```python
from build123d import *

# Parameters (mm, degrees)
SKETCH1_R           = 31.75
SKETCH1_R_2         = 29.21
BOSS_EXTRUDE1_DEPTH = 12.7
SKETCH2_W           = 76.2
SKETCH2_H           = 76.2
BOSS_EXTRUDE2_DEPTH = 2.54
FILLET1_R           = 6.35


with BuildPart() as part:
    # Sketch1 → Boss-Extrude1 (new body)
    with BuildSketch(Plane(origin=(0, 0, 0), x_dir=(1, 0, 0), z_dir=(0, 1, 0))):
        with Locations(Location((0, 0, 0), (0, 0, 270))):
            Circle(SKETCH1_R)
        with Locations(Location((0, 0, 0), (0, 0, 270))):
            Circle(SKETCH1_R_2, mode=Mode.SUBTRACT)
    extrude(amount=BOSS_EXTRUDE1_DEPTH)

    # Sketch2 → Boss-Extrude2 (add)
    with BuildSketch(Plane(origin=(0, 0, 0), x_dir=(1, 0, 0), z_dir=(0, 1, 0))):
        Rectangle(SKETCH2_W, SKETCH2_H)
    extrude(amount=BOSS_EXTRUDE2_DEPTH)

    # Fillet1
    fillet1_edges = [part.edges().sort_by_distance(p)[0] for p in [
        (38.1, 1.27, 38.1),
        (38.1, 1.27, -38.1),
        (-38.1, 1.27, -38.1),
        (-38.1, 1.27, 38.1),
    ]]
    fillet(fillet1_edges, radius=FILLET1_R)


solid = part.part
```
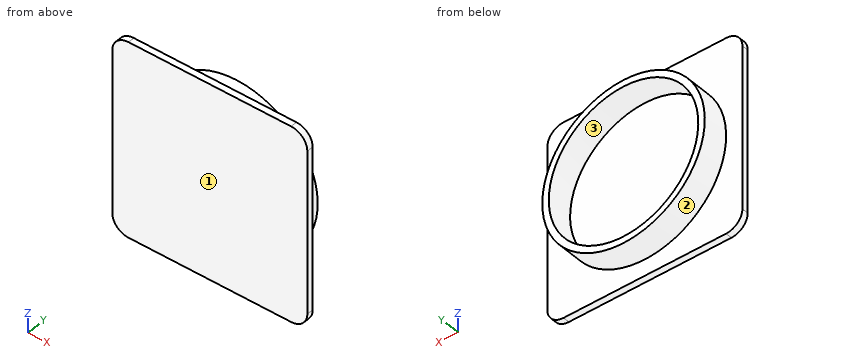
The model under review builds one solid part; all positions refer to its coordinate system, in mm. Face numbers are marked on the shaded views. Round coordinates to 2 decimals unless told otherwise and drop trailing zeros. Loops run counter-clockwise (first coordinate to the right, second up) from the corner with the lowest first, then second, coordinate; pieces in that order, holes last. Notation, with made-up numbers: (84, 75) - (105, 75) arc R17 cw to (105, 100) - close; hole circle Ø2 at (14.25, -36). An arc over 180 degrees is marked (long way). Use a Markdown table: item, result. Add a question column.
Q1. Insertion check: pin 1 Ø2 at (x, z) = (18.5, 0) entering from +Y; pin 2 Ø3 at (y, z) = (6.5, 1) entering from +X. Each pin has a flat end and moves straight along its axis. Give the tip position at first contact, or say it passes through.
Q2. Add section C-C (y = 6.5). State the section outline as (x, z) points, plus the area to 3 significant figures.
Q3. For probe 1 along X at (y, z) = (9, 0); probe 2 along Y at (x, z) = (-19.5, -3), list the stretches that pass through material, from the lowest coordinate up.
Q4. Add section A-A (x = 0). State the section outline as (y, z) points, plus the area to 3 significant figures.
Q5. The part is to be moulded in two halves that separate along Z. For the marked faces 1, 2 and 3, say which applies: pulls with the +Z half, pulls with the -Z half, needs draft (parallel to the pull), parting line crosses it, or undercut.
Q6. Add section B-B (z = 0). State the section outline as (x, y) points, plus the area to 3 significant figures.
Worked answers:
| question | item | result |
|---|---|---|
| 1 | pin 1 | y = 2.54 |
| 1 | pin 2 | x = 31.75 |
| 2 | outline | circle Ø63.5 at (0, 0); hole circle Ø58.42 at (0, 0) |
| 2 | area | 486 mm² |
| 3 | probe 1 | -31.75 to -29.21, 29.21 to 31.75 |
| 3 | probe 2 | 0 to 2.54 |
| 4 | outline | (0, -38.1) - (2.54, -38.1) - (2.54, -31.75) - (12.7, -31.75) - (12.7, -29.21) - (2.54, -29.21) - (2.54, 29.21) - (12.7, 29.21) - (12.7, 31.75) - (2.54, 31.75) - (2.54, 38.1) - (0, 38.1) - close |
| 4 | area | 245 mm² |
| 5 | face 1 | needs draft |
| 5 | face 2 | parting line crosses it |
| 5 | face 3 | undercut |
| 6 | outline | (-38.1, 0) - (38.1, 0) - (38.1, 2.54) - (31.75, 2.54) - (31.75, 12.7) - (29.21, 12.7) - (29.21, 2.54) - (-29.21, 2.54) - (-29.21, 12.7) - (-31.75, 12.7) - (-31.75, 2.54) - (-38.1, 2.54) - close |
| 6 | area | 245 mm² |
